Part model, mm, in its own coordinate system. Face numbers are marked on the shaded views. A direction names the side the tool comes from. Coordinates: 2 decimals unless noted, no trailing zeros. Write each loop counter-clockwise with the first axis right and the second up, starting at its lowest first coordinate (ties: lowest second). Pieces come first, ordered by that corner, then holes. Notation, with made-up numbers: (11.25, 31.5) - (39.25, 31.5) arc R25 ccw to (39.25, 57.5) - close; hole circle Ø11 at (-21, 84). An arc over 180 degrees is marked (long way). Use a Markdown table: item, result.
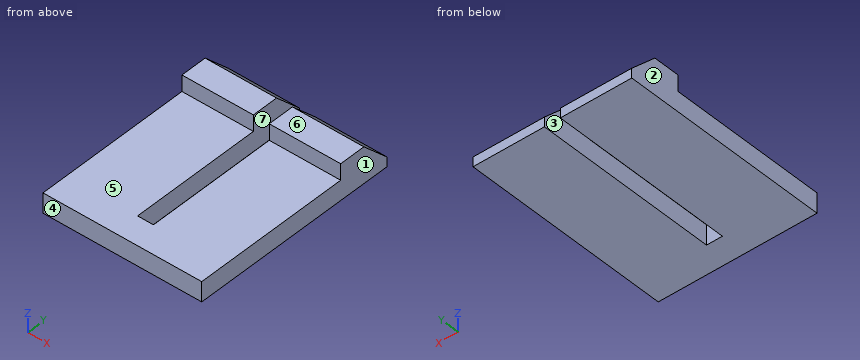
```python
from build123d import *

# Parameters (mm, degrees)
F0_W     = 13.5
F0_H     = 25
F0_W_2   = 1.5
F0_H_2   = 5
F1_DEPTH = 3.75
F0_H_3   = 10
F2_DEPTH = 6.8
F3_SIZE  = 5


with BuildPart() as f1:
    # F0 (on Top) → F1 (new body)
    with BuildSketch(Plane.XY):
        with Locations((-8.25, 17.5)):
            Rectangle(F0_W, F0_H)
        Polygon((1.5, 30), (1.5, 5), (15, 4.9196085972), (15, 30), align=None)
        Polygon((1.5, 5), (1.5, 0), (15, 0), (15, 4.9196085972), align=None)
        with Locations((0.75, 2.5)):
            Rectangle(F0_W_2, F0_H_2)
        with Locations((-0.75, 2.5)):
            Rectangle(F0_W_2, F0_H_2)
        with Locations((-8.25, 2.5)):
            Rectangle(F0_W, F0_H_2)
    extrude(amount=F1_DEPTH)

    # F0 (on Top) → F2 (join)
    with BuildSketch(Plane.XY):
        with Locations((-8.25, 35)):
            Rectangle(F0_W, F0_H_3)
        with Locations((8.25, 35)):
            Rectangle(F0_W, F0_H_3)
    extrude(amount=F2_DEPTH)

    # F3
    f3_edges = [f1.edges().sort_by_distance(p)[0] for p in [
        (-8.25, 40, 6.8),
        (8.25, 40, 6.8),
    ]]
    chamfer(f3_edges, length=F3_SIZE)


solid = f1.part
```
Item 1: Band-saw the part on C-C, the plane z = 0.5. Give the cut face in (x, y).
From the geometry:
| item | result |
|---|---|
| outline | (-15, 0) - (15, 0) - (15, 40) - (1.5, 40) - (1.5, 5) - (-1.5, 5) - (-1.5, 40) - (-15, 40) - close |
Item 2: Drill centre lines: probe 1 along X at (y, z) = (38, 1); probe 2 along Z at (x, y) = (-7.75, 4); probe 3 along Y at (x, z) = (0.5, 3). Where is each one in solid material? Low to high.
From the geometry:
| item | result |
|---|---|
| probe 1 | -15 to -1.5, 1.5 to 15 |
| probe 2 | 0 to 3.75 |
| probe 3 | 0 to 5 |
Item 3: Which spindle directions (+Z, -Z, +X, -X, +Y, -Y) get a long thin tool onto all of the face, cutting with end or side? Do the marked faces 5, 6 and 7. Say none if no direction does.
From the geometry:
| item | result |
|---|---|
| face 5 | +Z, +X, -X, -Y |
| face 6 | +Z, +X, -X, +Y, -Y |
| face 7 | +Z, -Z, +Y |
Item 4: Drop flat-ended pins along their axis: P1, Ø3, axis at x = -8, z = 4.5, coming from the +Y side; P2, Ø3.5, axis at x = 5, z = 6, coming from the -Y side; P3, Ø0.9, axis at x = 0, z = 2.5, coming from the +Y side. Give the stop position or say it passes through.
From the geometry:
| item | result |
|---|---|
| P1 | y = 38.8 |
| P2 | y = 30 |
| P3 | y = 5 |
Item 5: Two-plate mould, pull along X, no slides. Class the marked faces 1, 2, 3 and 4: pulls with the +X half, pulls with the -X half, needs draft (parallel to the pull), parting line crosses it, or undercut.
From the geometry:
| item | result |
|---|---|
| face 1 | pulls with the +X half |
| face 2 | pulls with the -X half |
| face 3 | undercut |
| face 4 | needs draft |
Item 6: Band-saw the part on D-D, the plane y = 16. Give the cut face in (x, z), then the cut area to 3 significant figures.
From the geometry:
| item | result |
|---|---|
| outline | (-15, 0) - (-1.5, 0) - (-1.5, 3.75) - (-15, 3.75) - close; (1.5, 0) - (15, 0) - (15, 3.75) - (1.5, 3.75) - close |
| area | 101 mm^2 |
Item 7: Band-saw the part on B-B, the plane x = 13. Give the cut face in (y, z), then the cut area to 3 significant figures.
From the geometry:
| item | result |
|---|---|
| outline | (0, 0) - (40, 0) - (40, 1.8) - (35, 6.8) - (30, 6.8) - (30, 3.75) - (0, 3.75) - close |
| area | 168 mm^2 |
Item 8: Band-saw the part on A-A, the plane y = 32. Give the cut face in (x, z).
From the geometry:
| item | result |
|---|---|
| outline | (-15, 0) - (-1.5, 0) - (-1.5, 6.8) - (-15, 6.8) - close; (1.5, 0) - (15, 0) - (15, 6.8) - (1.5, 6.8) - close |
